Can you work these out from the model? Positions are in its coordinate system, mm. A direction names the side the tool comes from. Coordinates: 2 decimals unless noted, no trailing zeros. Write each loop counter-clockwise with the first axis right and the second up, starting at its lowest first coordinate (ties: lowest second). Pieces come first, ordered by that corner, then holes. Notation, with made-up numbers: (49, -24) - (75, -24) arc R25 ccw to (75, 2) - close; hole circle Ø11 at (59, 70.25). An arc over 180 degrees is marked (long way). Use one line per item in the form item = value. Start each with the question number.
(1) Thinking about a two-plate mould opening in Y: for faces 4 (the face through (27, -33, 10)), 5 (the face through (-43, 13, 10)), 6 (the face through (-26.3, 57.4, 20)), which applies, pulls with the +Y half, pulls with the -Y half, needs draft (parallel to the pull), parting line crosses it, or undercut?
(2) If we section it at B-B on z = 12: Please give me the cut outline in (x, y).
(3) On a 3-axis mill with a long thin cutter (end or side, diameter ignored), from which of +Z, -Z, +X, -X, +Y, -Y can I reach the whole of each face in a straight line? I mean faces 1 (the face through (-26, -33, -10)), 2 (the face through (-26.3, 57.4, -20)), 3 (the face through (0, 45, 10)). Say none if no direction works.
(4) For pin 1 Ø8 at (y, z) = (-44.5, -6.5) entering from +X; pin 2 Ø8 at (x, y) = (45, 12) entering from -Z; pin 3 Ø6 at (x, z) = (-2, 10) entering from +Y; pin 4 Ø6.5 at (x, y) = (0, 0) entering from +Z, each with a flat end and sliding along its axis, tell me the tip position at first contact or that it passes through.
(5) If I drill on probe 1 along Y at (x, z) = (0, -4); probe 2 along Y at (x, z) = (0, -16.75); probe 3 along X at (y, z) = (-6.5, -7), over which ranges is the centre line in solid material (lowest first)? Write a range as from..to.
(6) If we section it at C-C on y = 46.5: Give the number of separate pieces and of enclosed holes in the cut face, then the cut area to 3 significant figures.
(7) If we section it at A-A on x = 0: Please give me the cut outline in (y, z), then the cut area to 3 significant figures.
```python
from build123d import *

# Parameters (mm, degrees)
SKETCH1_R           = 70
SKETCH1_R_2         = 62.278635001
SKETCH1_R_3         = 17.121532135
SKETCH1_R_4         = 4
BOSS_EXTRUDE1_DEPTH = 20
SKETCH2_R           = 62.5
SKETCH2_R_2         = 17.5
CUT_EXTRUDE1_DEPTH  = 10
CUT_EXTRUDE2_DEPTH  = 104.440804328


with BuildPart() as part:
    # Sketch1 → Boss-Extrude1 (new, symmetric)
    # profile 1 of 3: a face of its own
    with BuildSketch(Plane.XY):
        Circle(SKETCH1_R)
        Circle(SKETCH1_R_2, mode=Mode.SUBTRACT)
    # profile 2 of 3: a face of its own
    with BuildSketch(Plane.XY):
        Circle(SKETCH1_R_2)
        Circle(SKETCH1_R_3, mode=Mode.SUBTRACT)
    # profile 3 of 3: a face of its own
    with BuildSketch(Plane.XY):
        Circle(SKETCH1_R_3)
        Circle(SKETCH1_R_4, mode=Mode.SUBTRACT)
    extrude(amount=BOSS_EXTRUDE1_DEPTH, both=True)

    # Sketch2 → Cut-Extrude1 (cut)
    with BuildSketch(Plane(origin=(0, 0, -20), x_dir=(-1, 0, 0), z_dir=(0, 0, -1))):
        Circle(SKETCH2_R)
        Circle(SKETCH2_R_2, mode=Mode.SUBTRACT)
    cut_extrude1 = extrude(amount=-CUT_EXTRUDE1_DEPTH, mode=Mode.SUBTRACT)

    # Mirror1: Cut-Extrude1 across plane
    add(cut_extrude1.mirror(Plane.XY), mode=Mode.SUBTRACT)

    # Sketch3 → Cut-Extrude2 (cut, through all)
    with BuildSketch(Plane(origin=(0, 0, -10), x_dir=(-1, 0, 0), z_dir=(0, 0, -1))):
        with BuildLine():
            add(Edge.make_bspline(
                [(-16.012184604, 60.414070747), (-10.028198069, 38.589231507), (-6.603566708, 16.206261343)],
                knots=[0, 0, 0, 1, 1, 1], degree=2))
            ThreePointArc((-16.012184604, 60.414070747), (-36.736578268, 50.563562148), (-52.5091585, 33.897467068))
            add(Edge.make_bspline(
                [(-52.5091585, 33.897467068), (-33.601656457, 21.462111455), (-13.372456119, 11.288375319)],
                knots=[0, 0, 0, 1, 1, 1], degree=2))
            ThreePointArc((-13.372456119, 11.288375319), (-10.286241915, 14.157797402), (-6.603566708, 16.206261343))
        make_face()
        with BuildLine():
            add(Edge.make_bspline(
                [(52.5091585, 33.897467068), (33.601656457, 21.462111455), (13.372456119, 11.288375319)],
                knots=[0, 0, 0, 1, 1, 1], degree=2))
            ThreePointArc((52.5091585, 33.897467068), (36.736578268, 50.563562148), (16.012184604, 60.414070747))
            add(Edge.make_bspline(
                [(16.012184604, 60.414070747), (10.028198069, 38.589231507), (6.603566708, 16.206261343)],
                knots=[0, 0, 0, 1, 1, 1], degree=2))
            ThreePointArc((6.603566708, 16.206261343), (10.286241915, 14.157797402), (13.372456119, 11.288375319))
        make_face()
        with BuildLine():
            ThreePointArc((48.464629278, -39.464283966), (58.886710427, -20.942906557), (62.5, 0))
            ThreePointArc((62.5, 0), (62.476303713, 1.720893487), (62.405232819, 3.440482052))
            add(Edge.make_bspline(
                [(62.405232819, 3.440482052), (39.79942371, 2.387345216), (17.453684792, -1.272354978)],
                knots=[0, 0, 0, 1, 1, 1], degree=2))
            ThreePointArc((17.453684792, -1.272354978), (16.643489035, -5.407797402), (14.868199103, -9.229661719))
            add(Edge.make_bspline(
                [(48.464629278, -39.464283966), (30.795163838, -25.324917157), (14.868199103, -9.229661719)],
                knots=[0, 0, 0, 1, 1, 1], degree=2))
        make_face()
        with BuildLine():
            ThreePointArc((-62.405232819, 3.440482052), (-59.441032268, -19.313562148), (-48.464629278, -39.464283966))
            add(Edge.make_bspline(
                [(-48.464629278, -39.464283966), (-30.795163838, -25.324917157), (-14.868199103, -9.229661719)],
                knots=[0, 0, 0, 1, 1, 1], degree=2))
            ThreePointArc((-14.868199103, -9.229661719), (-16.643489035, -5.407797402), (-17.453684792, -1.272354978))
            add(Edge.make_bspline(
                [(-62.405232819, 3.440482052), (-39.79942371, 2.387345216), (-17.453684792, -1.272354978)],
                knots=[0, 0, 0, 1, 1, 1], degree=2))
        make_face()
        with BuildLine():
            ThreePointArc((-22.556370354, -58.287735901), (0, -62.5), (22.556370354, -58.287735901))
            add(Edge.make_bspline(
                [(22.556370354, -58.287735901), (14.569198516, -37.113771021), (4.183403722, -16.992619966)],
                knots=[0, 0, 0, 1, 1, 1], degree=2))
            ThreePointArc((4.183403722, -16.992619966), (0, -17.5), (-4.183403722, -16.992619966))
            add(Edge.make_bspline(
                [(-22.556370354, -58.287735901), (-14.569198516, -37.113771021), (-4.183403722, -16.992619966)],
                knots=[0, 0, 0, 1, 1, 1], degree=2))
        make_face()
    extrude(amount=-CUT_EXTRUDE2_DEPTH, mode=Mode.SUBTRACT)


solid = part.part
```
Reported:
q1.face_4 = undercut
q1.face_5 = undercut
q1.face_6 = needs draft
q2.outline = circle Ø140 at (0, 0); circle Ø35 at (0, 0); hole circle Ø125 at (0, 0); hole circle Ø8 at (0, 0)
q3.face_1 = -Z
q3.face_2 = -Z, +X, -X, +Y, -Y
q3.face_3 = +Z
q4.pin_1 = 57.09
q4.pin_2 = -10
q4.pin_3 = 70
q4.pin_4 = through
q5.probe_1 = -70..-62.5, -17.5..-4, 4..70
q5.probe_2 = -70..-62.5, -17.5..-4, 4..17.5, 62.5..70
q5.probe_3 = -69.7..-62.16, -16.25..16.25, 62.16..69.7
q6.separate_pieces = 3
q6.enclosed_holes = 0
q6.area = 1,340 mm2
q7.outline = (-70, -20) - (-62.5, -20) - (-62.5, 20) - (-70, 20) - close; (-17.5, -20) - (-4, -20) - (-4, 20) - (-17.5, 20) - close; (4, -20) - (17.5, -20) - (17.5, -10) - (62.5, -10) - (62.5, -20) - (70, -20) - (70, 20) - (62.5, 20) - (62.5, 10) - (17.5, 10) - (17.5, 20) - (4, 20) - close
q7.area = 2,580 mm2
